```python
from build123d import *

# Parameters (mm, degrees)
F0_W      = 787.4
F0_H      = 400.05
F1_DEPTH  = 241.3
F2_R      = 62.23
F3_DEPTH  = 50.8
F4_W      = 744.22
F4_H      = 356.87
F5_DEPTH  = 215.9
F6_R      = 82.55
F6_R_2    = 60.96
F7_DEPTH  = 215.9
F8_W      = 5.5862860754
F8_H      = 356.87
F9_DEPTH  = 154.94
F10_DEPTH = 254
F11_DEPTH = 154.94


with BuildPart() as f1:
    # F0 (on Top) → F1 (new body)
    with BuildSketch(Plane.XY):
        Rectangle(F0_W, F0_H)
    extrude(amount=F1_DEPTH)

    # F2 (on face) → F3 (join)
    with BuildSketch(Plane.XY.offset(241.3)):
        with Locations((-254.7448580774, -95.225625706)):
            Circle(F2_R)
        with Locations((-255.5709736083, 95.274374294)):
            Circle(F2_R)
        with Locations((-2.9369472516, 99.4085264267)):
            Circle(F2_R)
        with Locations((5.3922456924, -91.0914735733)):
            Circle(F2_R)
        with Locations((225.107953531, 95.9239800905)):
            Circle(F2_R)
        with Locations((228.7954458169, -94.5760199095)):
            Circle(F2_R)
    extrude(amount=F3_DEPTH)

    # F4 (on face) → F5 (cut)
    with BuildSketch(Plane(origin=(0, 0, 0), x_dir=(1, 0, 0), z_dir=(0, 0, -1))):
        Rectangle(F4_W, F4_H)
    extrude(amount=-F5_DEPTH, mode=Mode.SUBTRACT)

    # F6 (on face) → F7 (join)
    with BuildSketch(Plane(origin=(0, 0, 215.9), x_dir=(1, 0, 0), z_dir=(0, 0, -1))):
        with Locations((-252.7241706848, 0)):
            Circle(F6_R)
        with Locations((-252.7241706848, 0)):
            Circle(F6_R_2, mode=Mode.SUBTRACT)
        Circle(F6_R)
        Circle(F6_R_2, mode=Mode.SUBTRACT)
        with Locations((252.73, 0)):
            Circle(F6_R)
        with Locations((252.73, 0)):
            Circle(F6_R_2, mode=Mode.SUBTRACT)
    extrude(amount=F7_DEPTH)

    # F8 (on face) → F9 (join)
    with BuildSketch(Plane(origin=(0, 0, 215.9), x_dir=(1, 0, 0), z_dir=(0, 0, -1))):
        Rectangle(F8_W, F8_H)
    extrude(amount=F9_DEPTH)

    # F10 (cut): faces of the model
    f10_faces = [f1.faces().sort_by_distance(p)[0] for p in [
        (-27.3880241928, 0, 215.9),
        (27.3880241928, 0, 215.9),
    ]]
    extrude(f10_faces, amount=F10_DEPTH, mode=Mode.SUBTRACT)

    # F11 (cut): a face of the model
    f11_faces = [f1.faces().sort_by_distance(p)[0] for p in [
        (0, 0, 60.96),
    ]]
    extrude(f11_faces, amount=-F11_DEPTH, mode=Mode.SUBTRACT)


solid = f1.part
```
Build history of the part. All positions in model axes, mm. A direction names the side the tool comes from. Give positions to 0.01 mm unless a question says otherwise; leave off trailing zeros. Loops run counter-clockwise (first coordinate to the right, second up) from the corner with the lowest first, then second, coordinate; pieces in that order, holes last. Notation, with made-up numbers: (-6.5, 83.5) -> (36.5, 83.5) arc R15 cw to (36.5, 108.5) -> close; hole circle Ø9 at (-33.5, 63). An arc over 180 degrees is marked (long way). One line per question, with ' | ' between items. Start each with the question number.
1) Cut at D-D (z = 269.5). Give the cut face in (x, y).
2) Cut at A-A (z = 163). Give the cut face in (x, y) (3 decimals), plus the area to 3 significant figures.
3) Two-plate mould, pull along X, no slides. Class faces 4 (the cylindrical face through (191.83, -2.68, 109.46)), 5 (the flat face through (-149, -2, 215.9)), 6 (the flat face through (-393.7, -3, 119)), 7 (the flat face through (224, 97, 292.1)): released by +X, released by -X, zero draft, split by the parting line, or undercut.
4) 3-axis set-ups, long thin cutter, end or side, ignore diameter. For faces 1 (the flat face through (-372.11, 2, 106)), 2 (the cylindrical face through (-16.43, 38.66, 266.34)), 3 (the flat face through (-259, 61, 0)): which of +Z, -Z, +X, -X, +Y, -Y reach the whole face in a straight line?
5) Pin check, flat tips, straight feed: pin 1 (1.7 mm diameter, centred on x = 0.5, y = 141, fed in from -Z); pin 2 (6 mm diameter, centred on x = 61.5, y = -40, fed in from +Z); pin 3 (5 mm diameter, centred on x = 103, y = -56, fed in from -Z). Stop position of each tip, or through.
6) Cut at C-C (x = 252.73). Give the cut face in (y, z) (3 decimals).
7) Probe L1, parallel to X at y = 113, z = 104; L2, parallel to Y at x = 252.73, z = 137 (3 decimals); L3, parallel to Y at x = 0, z = 145 (3 decimals). List the from-to ranges inside material, lowest first.
Return value:
1) outline: circle Ø124.46 at (-255.57, 95.27); circle Ø124.46 at (-254.74, -95.23); circle Ø124.46 at (-2.94, 99.41); circle Ø124.46 at (5.39, -91.09); circle Ø124.46 at (225.11, 95.92); circle Ø124.46 at (228.8, -94.58)
2) outline: (-393.7, -200.025) -> (393.7, -200.025) -> (393.7, 200.025) -> (-393.7, 200.025) -> close; circle Ø165.1 at (-252.724, 0); circle Ø165.1 at (252.73, 0); hole (-372.11, -178.435) -> (-2.793, -178.435) -> (-2.793, -82.503) arc R82.55 cw to (-2.793, 82.503) -> (-2.793, 178.435) -> (-372.11, 178.435) -> close; hole circle Ø121.92 at (-252.724, 0); hole circle Ø121.92 at (0, 0); hole (2.793, -178.435) -> (372.11, -178.435) -> (372.11, 178.435) -> (2.793, 178.435) -> (2.793, 82.503) arc R82.55 cw to (2.793, -82.503) -> close; hole circle Ø121.92 at (252.73, 0) | area: 79,700 mm^2
3) face 4: undercut | face 5: undercut | face 6: released by -X | face 7: zero draft
4) face 1: -Z | face 2: +Z | face 3: -Z, +X, -X, +Y, -Y
5) pin 1: z = 60.96 | pin 2: z = 241.3 | pin 3: z = 215.9
6) outline: (-200.025, 0) -> (-178.435, 0) -> (-178.435, 215.9) -> (-82.55, 215.9) -> (-82.55, 0) -> (-60.96, 0) -> (-60.96, 215.9) -> (60.96, 215.9) -> (60.96, 0) -> (82.55, 0) -> (82.55, 215.9) -> (178.435, 215.9) -> (178.435, 0) -> (200.025, 0) -> (200.025, 241.3) -> (151.688, 241.3) -> (151.688, 292.1) -> (40.16, 292.1) -> (40.16, 241.3) -> (-37.133, 241.3) -> (-37.133, 292.1) -> (-152.019, 292.1) -> (-152.019, 241.3) -> (-200.025, 241.3) -> close
7) L1: -393.7 to -372.11, -2.79 to 2.79, 372.11 to 393.7 | L2: -200.025 to -178.435, -82.55 to -60.96, 60.96 to 82.55, 178.435 to 200.025 | L3: -200.025 to -60.96, 60.96 to 200.025
